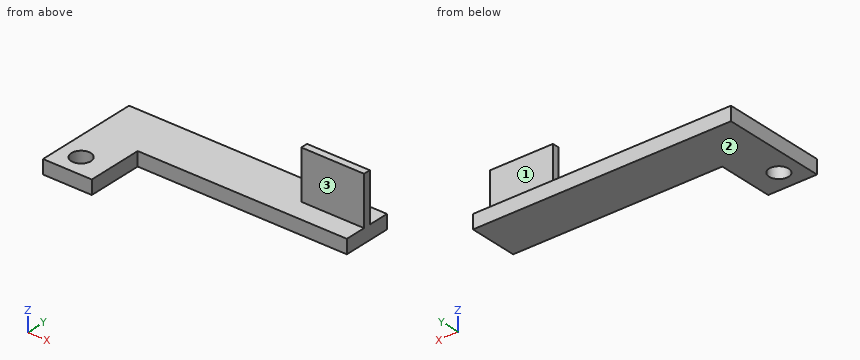
Autodesk Fusion 360 part; units mm, degrees
sketch "Sketch1" plane through (0, 0, 0) normal (0, 0, 1) x (1, 0, 0)
  line L0 (16.5, -3.5) -> (-16.5, -3.5)
  line L1 (-16.5, -3.5) -> (-16.5, 3.5)
  line L2 (-16.5, 3.5) -> (16.5, 3.5)
  line L3 (16.5, 3.5) -> (16.5, -3.5)
  line L4 (16.5, -3.5) -> (-16.5, 3.5) construction
  line L5 (-16.5, -3.5) -> (16.5, 3.5) construction
  circle A0 centre (-13.5, -8.5) radius 1.4
  line L6 (-16.5, 3.5) -> (-9.5, 3.5)
  line L7 (-9.5, 3.5) -> (-9.5, -11.5)
  line L8 (-9.5, -11.5) -> (-16.5, -11.5)
  line L9 (-16.5, -11.5) -> (-16.5, 3.5)
  dimension "d1" = 33
  dimension "d2" = 7
  dimension "d3" = 2.8
  dimension "d4" = 3
  dimension "d16" = 15
  dimension "d17" = 3
  dimension "d18" = 7
extrude "Extrude1" add sketch "Sketch1" along normal blind 2
sketch "Sketch2" plane through (16.5, 0, 0) normal (1, 0, 0) x (0, 1, 0)
  line L0 (-3.5, 0) -> (3.5, 0)
  line L1 (3.5, 0) -> (3.5, 2)
  line L2 (3.5, 2) -> (-3.5, 2)
  line L3 (-3.5, 2) -> (-3.5, 0)
  line L4 (0, 2) -> (0.5, 2)
  line L5 (0.5, 2) -> (0.5, 12)
  line L6 (0.5, 12) -> (0, 12)
  line L7 (0, 12) -> (0, 2)
  line L8 (0, 12) -> (-0.5, 12)
  line L9 (-0.5, 12) -> (-0.5, 2)
  line L10 (-0.5, 2) -> (0, 2)
  line L11 (0, 2) -> (0, 12)
  dimension "d7" = 0.5
  dimension "d8" = 10
  dimension "d9" = 0.5
extrude "Extrude2" add sketch "Sketch2" against normal blind 5 contours L2 L7 L8 L9 L10 L11 | L2 L4 L5 L6 L7 L11
extrude "Extrude3" add 1 faces at (16.5, 0.1667, 0.6667) along direction (1, 0, 0) blind 4
extrude "Extrude4" cut 1 faces at (17.5, -0.1667, 12) along direction (0, 0, -1) blind 3
equation "d1 = 25 mm + 8 mm"
Could you check a few things on this model? Use its own coordinates, in mm. Face numbers are marked on the shaded views. A direction names the side the tool comes from. Round coordinates to 2 decimals unless told otherwise and drop trailing zeros. Order: outer loops, then holes, each group sorted by start corner. A loop starts at its lowest first (then second) coordinate and runs counter-clockwise, first axis right, second up. Notation, with made-up numbers: M 3.5,30.5 L 45.5,30.5 A24 cw 45.5,45.5 Z; hole C 8,-22 d9. An arc over 180 degrees is marked long. One line per question, with ' | ' between items. Start each with the question number.
(1) Please list where these lines run through material, in increasing order: line 1 along Y through (x, z) = (-13.5, 1.4); line 2 along Z through (x, y) = (-4.5, -3.25); line 3 along Y through (x, z) = (8, 0.5).
(2) For P1, Ø1.6, axis at x = 2, z = 0.5, coming from the -Y side; P2, Ø2, axis at y = -8, z = 1.5, coming from the +X side; P3, Ø2, axis at x = 15.5, z = 6.5, coming from the +Y side; P4, Ø5, axis at x = -9, z = 5, coming from the +Y side, each with a flat end and sliding along its axis, tell me the tip position at first contact or that it passes through.
(3) Suppose I cut it at A-A on y = -8.5. List the corners of the cut face in (x, z) for me, then the cut area to 3 significant figures.
(4) For the marked faces 1, 2 and 3, which set-ups out of +Z, -Z, +X, -X, +Y, -Y let a thin tool reach every point of the face, with its end or its side?
(5) Suppose I cut it at C-C on z = 1. List the corners of the cut face in (x, y) for me, then the cut area to 3 significant figures.
(6) Suppose I cut it at D-D on x = 14. List the corners of the cut face in (y, z) for me, then the cut area to 3 significant figures.
(7) Suppose I cut it at B-B on x = -13.5. List the corners of the cut face in (y, z) for me.
Geometry results:
1) line 1: -11.5 to -9.9, -7.1 to 3.5 | line 2: 0 to 2 | line 3: -3.5 to 3.5
2) P1: y = -3.5 | P2: x = -9.5 | P3: y = 0.5 | P4: through
3) outline: M -16.5,0 L -14.9,0 L -14.9,2 L -16.5,2 Z; M -12.1,0 L -9.5,0 L -9.5,2 L -12.1,2 Z | area: 8.40 mm²
4) face 1: +Z, +X, -X, +Y | face 2: -Z, +X, -X, +Y, -Y | face 3: +Z, +X, -X, -Y
5) outline: M -16.5,-11.5 L -9.5,-11.5 L -9.5,-3.5 L 20.5,-3.5 L 20.5,3.5 L -16.5,3.5 Z; hole C -13.5,-8.5 d2.8 | area: 309 mm²
6) outline: M -3.5,0 L 3.5,0 L 3.5,2 L 0.5,2 L 0.5,9 L -0.5,9 L -0.5,2 L -3.5,2 Z | area: 21.0 mm²
7) outline: M -11.5,0 L -9.9,0 L -9.9,2 L -11.5,2 Z; M -7.1,0 L 3.5,0 L 3.5,2 L -7.1,2 Z
